Read the model definition and answer for the solid it produces. Units are mm, in the model's axes. A direction names the side the tool comes from. Give positions to 0.01 mm unless a question says otherwise; leave off trailing zeros. Order: outer loops, then holes, each group sorted by start corner. A loop starts at its lowest first (then second) coordinate and runs counter-clockwise, first axis right, second up. Notation, with made-up numbers: (21, -28.75) - (69, -28.75) arc R19 ccw to (69, -5.75) - close; hole circle Ø9 at (38, -9). An arc over 180 degrees is marked (long way). Write item = value, one per line.
```python
from build123d import *

# Parameters (mm, degrees)
F0_R     = 5.08
F1_DEPTH = 11.684
F4_R     = 2.921
F5_DEPTH = 59.944
F6_R     = 2.38125
F7_DEPTH = 19.05


with BuildPart() as f1:
    # F0 (on Front) → F1 (new body)
    with BuildSketch(Plane.XZ):
        Circle(F0_R)
    extrude(amount=F1_DEPTH)

    # F2 (on Right) → F3 (revolve)
    with BuildSketch(Plane.YZ):
        with BuildLine():
            ThreePointArc((-18.796, -7.366), (-13.5874514498, -5.2085485502), (-11.43, 0))
            ThreePointArc((-11.43, 0), (-13.5874514498, 5.2085485502), (-18.796, 7.366))
            Line((-18.796, 7.366), (-18.796, 0))
            Line((-18.796, 0), (-18.796, -7.366))
        make_face()
    revolve(axis=Axis((0, -18.796, 0), (0, 0, -1)))

    # F4 (on face) → F5 (join)
    with BuildSketch(Plane(origin=(0, 0, 0), x_dir=(-1, 0, 0), z_dir=(0, 1, 0))):
        Circle(F4_R)
    extrude(amount=F5_DEPTH)

    # F6 (on Right) → F7 (join)
    with BuildSketch(Plane.YZ):
        with Locations((-19.558, 0)):
            Circle(F6_R)
    extrude(amount=F7_DEPTH)


solid = f1.part
```
1. Straight lines are drawn through the part: L1, parallel to Y at x = 0, z = -4.5; L2, parallel to Y at x = -4, z = -3; L3, parallel to Y at x = -3.25, z = 6. For each, find the intervals that lie inside material, in ascending order. Write a range as [from, to].
Recorded:
L1 = [-24.63, -12.96], [-11.68, 0]
L2 = [-24.21, -13.39], [-11.68, 0]
L3 = [-21.57, -16.02]
2. Section B-B (y = 20.5) is taken. Determine the outline of the cut face in (x, z).
Recorded:
outline = circle Ø5.84 at (0, 0)
3. Section D-D (z = -1) is taken. Determine the outline of the cut face in (x, y), and give its area (3 significant figures).
Recorded:
outline = (-4.98, -11.68) - (-1.64, -11.68) arc R7.3 ccw (long way) to (6.69, -21.72) - (19.05, -21.72) - (19.05, -17.4) - (7.16, -17.4) arc R7.3 ccw to (1.64, -11.68) - (4.98, -11.68) - (4.98, 0) - (2.74, 0) - (2.74, 59.94) - (-2.74, 59.94) - (-2.74, 0) - (-4.98, 0) - close
area = 664 mm^2
4. For faces 1 (the face through (19.05, -20, 0)), 2 (the face through (-0.661, -5.76, 5.037)), determine the directions among +Z, -Z, +X, -X, +Y, -Y from which every point of the face is accessible in a straight line to the end or side of a thin tool.
Recorded:
face_1 = +Z, -Z, +X, +Y, -Y
face_2 = +Y
5. Section A-A (x = 4) is taken. Determine the outline of the cut face in (y, z), and give its area (3 significant figures).
Recorded:
outline = circle Ø12.37 at (-18.8, 0); (-11.68, -3.13) - (0, -3.13) - (0, 3.13) - (-11.68, 3.13) - close
area = 193 mm^2
6. Flat-ended cylindrical pins translate along their axes: pin 1 (6 mm diameter, centred on x = 16, z = -4, fed in from +Y); pin 2 (6 mm diameter, centred on x = 0.5, z = -6, fed in from -Y); pin 3 (5 mm diameter, centred on x = -4.5, z = 2, fed in from -Y). Find the tip coordinate at first contact, or state that the pin passes through.
Recorded:
pin_1 = -17.4
pin_2 = -25.51
pin_3 = -25.75
7. Determine the mould class of faces 3 (the face through (2.2, 0, -2.2)), 4 (the face through (2.2, -11.684, -1.1)), 5 (the face through (0.633, 29.552, -2.852)), 6 (the face through (12.77, -17.29, 0.72)) for opening direction Y: +Y half, -Y half, draft (parallel to the pull), parting line (faces both ways), or undercut.
Recorded:
face_3 = +Y half
face_4 = undercut
face_5 = draft
face_6 = parting line
8. Section C-C (x = -0.75) is taken. Determine the outline of the cut face in (y, z).
Recorded:
outline = (-11.68, -5.02) - (0, -5.02) - (0, -2.82) - (59.94, -2.82) - (59.94, 2.82) - (0, 2.82) - (0, 5.02) - (-11.68, 5.02) - (-11.68, 1.76) arc R7.33 ccw (long way) to (-11.68, -1.76) - close
